```python
from build123d import *

# Parameters (mm, degrees)
F0_R      = 1.5
F0_R_2    = 1.6
F1_DEPTH  = 5
F2_R      = 3
F3_R      = 2
F4_R      = 5
F5_R      = 5
F6_R      = 1.5
F7_DEPTH  = 25
F9_DEPTH  = 25
F10_R     = 2
F11_R     = 1.65
F12_DEPTH = 25
F14_DEPTH = 25


with BuildPart() as f1:
    # F0 (on Top) → F1 (new body)
    with BuildSketch(Plane.XY):
        with BuildLine():
            Line((-9.9999813339, 0.0193215341), (0, 0))
            Line((0, 0), (0.4539924878, 0))
            Line((0.4539924878, 0), (0.4539924878, 22.4998891728))
            Line((0.4539924878, 22.4998891728), (12.9539924878, 47.5548288056))
            Line((12.9539924878, 47.5548288056), (23.5864712774, 53.8304637924))
            Line((23.5864712774, 53.8304637924), (25.5346026442, 54.9803143218))
            ThreePointArc((25.5346026442, 54.9803143218), (26.8013490925, 62.2870919693), (19.9533457596, 65.1328777146))
            Line((19.9533457596, 65.1328777146), (19.1141014773, 64.8209017638))
            Line((19.1141014773, 64.8209017638), (-2.4981679914, 56.7868782273))
            Line((-2.4981679914, 56.7868782273), (-40.5460603337, 56.7868782273))
            Line((-40.5460603337, 56.7868782273), (-61.6849283551, 64.8209017638))
            Line((-61.6849283551, 64.8209017638), (-62.7787610133, 65.2366230461))
            ThreePointArc((-62.7787610133, 65.2366230461), (-69.534777582, 62.3971715251), (-68.4220804384, 55.1536813523))
            Line((-68.4220804384, 55.1536813523), (-66.3019318016, 53.8657127229))
            Line((-66.3019318016, 53.8657127229), (-56.0460603337, 47.6353756185))
            Line((-56.0460603337, 47.6353756185), (-44.4999813339, 22.5804359857))
            Line((-44.4999813339, 22.5804359857), (-44.4999813339, 0))
            Line((-44.4999813339, 0), (-43.5460603337, 0))
            Line((-43.5460603337, 0), (-33.9999813339, 0.0656933026))
            Line((-33.9999813339, 0.0656933026), (-33.9999813339, 10.0656933026))
            Line((-33.9999813339, 10.0656933026), (-27.4999813339, 10.0656933026))
            Line((-27.4999813339, 10.0656933026), (-27.4999813339, 22.5656933026))
            Line((-27.4999813339, 22.5656933026), (-27.4999813339, 26.3816152201))
            Line((-27.4999813339, 26.3816152201), (-16.4999813339, 26.3816152201))
            Line((-16.4999813339, 26.3816152201), (-16.4999813339, 10.0656933026))
            Line((-16.4999813339, 10.0656933026), (-9.9999813339, 10.0656933026))
            Line((-9.9999813339, 10.0656933026), (-9.9999813339, 0.0193215341))
        make_face()
        with Locations((-4.888762403, 5.563379294)):
            Circle(F0_R, mode=Mode.SUBTRACT)
        with Locations((-55.4315750417, 55.6511066578)):
            Circle(F0_R_2, mode=Mode.SUBTRACT)
        with Locations((-60.4380198654, 57.9282781987)):
            Circle(F0_R_2, mode=Mode.SUBTRACT)
        with Locations((12.5329179775, 55.9733003324)):
            Circle(F0_R_2, mode=Mode.SUBTRACT)
        with Locations((17.6882422101, 57.8897115767)):
            Circle(F0_R_2, mode=Mode.SUBTRACT)
    extrude(amount=F1_DEPTH)

    # F2
    f2_edges = [f1.edges().sort_by_distance(p)[0] for p in [
        (-27.499981, 10.065693, 2.5),
        (-33.999981, 10.065693, 2.5),
        (-16.499981, 10.065693, 2.5),
        (-9.999981, 10.065693, 2.5),
        (-9.999981, 0.019322, 2.5),
        (-33.999981, 0.065693, 2.5),
        (-43.54606, 0, 2.5),
        (0.453992, 0, 2.5),
    ]]
    fillet(f2_edges, radius=F2_R)

    # F3
    f3_edges = [f1.edges().sort_by_distance(p)[0] for p in [
        (-16.499981, 26.381615, 2.5),
    ]]
    fillet(f3_edges, radius=F3_R)

    # F4
    f4_edges = [f1.edges().sort_by_distance(p)[0] for p in [
        (-43.54606, 0, 2.5),
        (0.453992, 22.499889, 2.5),
    ]]
    fillet(f4_edges, radius=F4_R)

    # F5
    f5_edges = [f1.edges().sort_by_distance(p)[0] for p in [
        (12.953992, 47.554829, 2.5),
        (-2.498168, 56.786878, 2.5),
        (-40.54606, 56.786878, 2.5),
        (-68.42208, 55.153681, 2.5),
        (-56.04606, 47.635376, 2.5),
    ]]
    fillet(f5_edges, radius=F5_R)

    # F6 (on face) → F7 (cut)
    with BuildSketch(Plane.XY.offset(5)):
        with Locations((-33.5573396883, 47.271139662)):
            Circle(F6_R)
        with Locations((-33.5573396883, 39.271139662)):
            Circle(F6_R)
        with Locations((-9.5573396883, 39.271139662)):
            Circle(F6_R)
        with Locations((-9.5573396883, 47.271139662)):
            Circle(F6_R)
    extrude(amount=-F7_DEPTH, mode=Mode.SUBTRACT)

    # F8 (on face) → F9 (cut)
    with BuildSketch(Plane.XY.offset(5)):
        Polygon((-16.7706497014, 48.1220260262), (-26.0973814875, 48.1220260262), (-27.693849057, 42.6604263484), (-27.693849057, 37.1988266706), (-15.0901572779, 37.1988266706), (-15.0901572779, 42.6604263484), align=None)
    extrude(amount=-F9_DEPTH, mode=Mode.SUBTRACT)

    # F10
    f10_edges = [f1.edges().sort_by_distance(p)[0] for p in [
        (-26.097381, 48.122026, 2.5),
        (-16.77065, 48.122026, 2.5),
        (-27.693849, 37.198827, 2.5),
        (-15.090157, 37.198827, 2.5),
    ]]
    fillet(f10_edges, radius=F10_R)

    # F11 (on face) → F12 (cut)
    with BuildSketch(Plane.XY.offset(5)):
        with Locations((-31.8884050022, 15.5689349914)):
            Circle(F11_R)
        with Locations((-12.1384050022, 15.5689349914)):
            Circle(F11_R)
        with Locations((-30.6362952974, 24.3189349914)):
            Circle(F11_R)
        with BuildLine():
            ThreePointArc((-11.241093269, 24.7316152201), (-13.0990926805, 26.368452489), (-14.4886523536, 24.3189349914))
            Line((-14.4886523536, 24.3189349914), (-11.2935341844, 24.3189349914))
            ThreePointArc((-11.2935341844, 24.3189349914), (-11.2542560001, 24.5236158086), (-11.241093269, 24.7316152201))
        make_face()
        with BuildLine():
            Line((-11.2935341844, 24.3189349914), (-14.4886523536, 24.3189349914))
            ThreePointArc((-14.4886523536, 24.3189349914), (-12.891093269, 23.0816152201), (-11.2935341844, 24.3189349914))
        make_face()
    extrude(amount=-F12_DEPTH, mode=Mode.SUBTRACT)

    # F13 (on face) → F14 (cut)
    with BuildSketch(Plane.XY.offset(5)):
        Polygon((-27.4999813339, 26.8493555486), (-27.4999813339, 24.3816152201), (-15.5926216394, 8.9839491993), (-15.5926216394, 26.8493555486), (-16.1031354219, 26.8493555486), align=None)
    extrude(amount=-F14_DEPTH, mode=Mode.SUBTRACT)


solid = f1.part
```
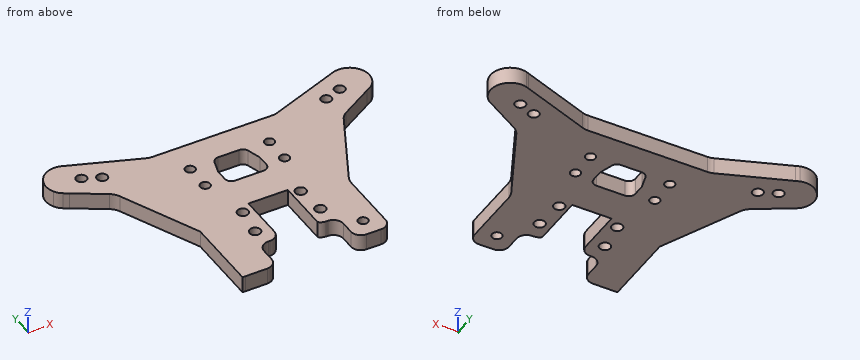
Could you check a few things on this model? Use its own coordinates, in mm. Give positions to 0.01 mm unless a question says otherwise; leave off trailing zeros. Order: outer loops, then holes, each group sorted by start corner. A loop starts at its lowest first (then second) coordinate and runs counter-clockwise, first axis right, second up.
Q1. Suppose I cut it at D-D, the plane x = 2.5. Write out the boundary of the cut face in (y, z).
Q2. I'm going to push flat-ended pins straight in: P1, Ø2.5, axis at y = 19.5, z = 1.5, coming from the +X side; P2, Ø2.5, axis at x = -20, z = 2.5, coming from the -Y side; P3, Ø1.5, axis at y = 15.5, z = 1.5, coming from the -X side. Where does each tip first touch, or does it pass through?
Q3. If I drill on line 1 along Y through (x, z) = (-19, 2.4); line 2 along X through (y, z) = (56, 3.2); line 3 along Y through (x, z) = (-12, 1.85), over which ranges is the centre line in solid material (lowest first)?
Q4. Suppose I cut it at A-A, the plane y = 20. Write out the boundary of the cut face in (x, z).
Q5. Suppose I cut it at B-B, the plane y = 12. Write out the boundary of the cut face in (x, z), and give its area (3 significant figures).
Q6. Suppose I cut it at C-C, the plane z = 1. Count the separate pieces of the cut face and the enclosed holes in it, and give its area (3 significant figures).
Solution:
1. outline: (26.6, 0) - (58.64, 0) - (58.64, 5) - (26.6, 5) - close
2. P1: stops at x = 0.45
2. P2: stops at y = 26.85
2. P3: stops at x = -44.5
3. line 1: y = 26.85 to 37.2, 48.12 to 56.79
3. line 2: x = -69.15 to -56.99, -53.87 to 10.93, 14.13 to 26.45
3. line 3: y = 9.89 to 13.92, 17.21 to 23.34, 26.12 to 56.79
4. outline: (-44.5, 0) - (-27.5, 0) - (-27.5, 5) - (-44.5, 5) - close; (-15.59, 0) - (0.45, 0) - (0.45, 5) - (-15.59, 5) - close
5. outline: (-44.5, 0) - (-27.7, 0) - (-27.7, 5) - (-44.5, 5) - close; (-15.59, 0) - (0.45, 0) - (0.45, 5) - (-15.59, 5) - close
5. area: 164 mm2
6. separate pieces: 1
6. enclosed holes: 14
6. area: 2,840 mm2
